The listing builds one solid part. Answer for the finished solid, in the listing's coordinates (mm). Give positions to 0.01 mm unless a question says otherwise; leave off trailing zeros. Loops run counter-clockwise (first coordinate to the right, second up) from the corner with the lowest first, then second, coordinate; pieces in that order, holes last. Notation, with made-up numbers: (27.5, 23) - (83.5, 23) arc R21 cw to (83.5, 59) - close; hole circle Ø7 at (86, -19.75). An arc over 180 degrees is marked (long way). Answer as CSV lines item,"result". Start each with the question number.
1) A flat-ended cylindrical pin translates along its axis: pin 1 (3 mm diameter, centred on y = -9.05, z = 15, fed in from +X). Find the tip coordinate at first contact, or state that the pin passes through.
2) A cutting plane is placed at C-C (z = 5.5). Determine the outline of the cut face in (x, y).
3) A cutting plane is placed at B-B (y = -54.05). Determine the outline of the cut face in (x, z), and give its area (3 significant figures).
4) For a pull along Z with two mould halves and no side action, classify faces 1 (the face through (27, -39, 1.59)), 2 (the face through (1.59, -39, 26)), 3 (the face through (25, -39, 0)), 4 (the face through (1, -9, 36)) as pulls with the +Z half, pulls with the -Z half, needs draft (parallel to the pull), parting line crosses it, or undercut.
5) A cutting plane is placed at D-D (y = -6). Determine the outline of the cut face in (x, z).
6) Find the intervals of material crossed by line 1 along Z through (x, y) = (0.85, -69.05); line 2 along Y through (x, z) = (0.9, 35); line 3 along X through (y, z) = (-30, 4), in increasing order.
7) A cutting plane is placed at A-A (z = 35). Determine the outline of the cut face in (x, y), and give its area (3 significant figures).
```python
from build123d import *

# Parameters (mm, degrees)
F1_DEPTH = 78.1
F2_R     = 1
F3_DEPTH = 50.801


with BuildPart() as f1:
    # F0 (on Front) → F1 (new body)
    with BuildSketch(Plane.XZ):
        Polygon((0, 50.8), (0, 0), (50.8, 0), (50.8, 1.59), (1.59, 1.59), (1.59, 50.8), align=None)
    extrude(amount=F1_DEPTH)

    # F2 (on Right) → F3 (cut, through all)
    with BuildSketch(Plane.YZ):
        with Locations((-9.05, 15)):
            Circle(F2_R)
        with Locations((-9.05, 35)):
            Circle(F2_R)
        with Locations((-24.05, 35)):
            Circle(F2_R)
        with Locations((-24.05, 15)):
            Circle(F2_R)
        with Locations((-54.05, 15)):
            Circle(F2_R)
        with Locations((-54.05, 35)):
            Circle(F2_R)
        with Locations((-69.05, 35)):
            Circle(F2_R)
        with Locations((-69.05, 15)):
            Circle(F2_R)
    extrude(amount=F3_DEPTH, mode=Mode.SUBTRACT)


solid = f1.part
```
Ans:
1,pin 1,"x = 1.59"
2,outline,"(0, -78.1) - (1.59, -78.1) - (1.59, 0) - (0, 0) - close"
3,outline,"(0, 0) - (50.8, 0) - (50.8, 1.59) - (1.59, 1.59) - (1.59, 14) - (0, 14) - close; (0, 16) - (1.59, 16) - (1.59, 34) - (0, 34) - close; (0, 36) - (1.59, 36) - (1.59, 50.8) - (0, 50.8) - close"
3,area,"153 mm2"
4,face 1,"pulls with the +Z half"
4,face 2,"needs draft"
4,face 3,"pulls with the -Z half"
4,face 4,"undercut"
5,outline,"(0, 0) - (50.8, 0) - (50.8, 1.59) - (1.59, 1.59) - (1.59, 50.8) - (0, 50.8) - close"
6,line 1,"0 to 14, 16 to 34, 36 to 50.8"
6,line 2,"-78.1 to -70.05, -68.05 to -55.05, -53.05 to -25.05, -23.05 to -10.05, -8.05 to 0"
6,line 3,"0 to 1.59"
7,outline,"(0, -78.1) - (1.59, -78.1) - (1.59, -70.05) - (0, -70.05) - close; (0, -68.05) - (1.59, -68.05) - (1.59, -55.05) - (0, -55.05) - close; (0, -53.05) - (1.59, -53.05) - (1.59, -25.05) - (0, -25.05) - close; (0, -23.05) - (1.59, -23.05) - (1.59, -10.05) - (0, -10.05) - close; (0, -8.05) - (1.59, -8.05) - (1.59, 0) - (0, 0) - close"
7,area,"111 mm2"
